```python
from build123d import *

# Parameters (mm, degrees)
SKETCH1_R                       = 72
SKETCH1_R_2                     = 60
BOSS_EXTRUDE1_DEPTH             = 25.4
BOSS_EXTRUDE4_DEPTH             = 12
CUT_EXTRUDE1_DEPTH              = 25.4
SKETCH8_W                       = 60
SKETCH8_H                       = 84.7705
BOSS_EXTRUDE5_DEPTH             = 12
CIRPATTERN4_COUNT               = 2
CIRPATTERN4_ANGLE               = 90
CIRPATTERN4_THE_OTHER_WAY_COUNT = 2
CIRPATTERN4_THE_OTHER_WAY_ANGLE = 90
M8_CLEARANCE_HOLE1_D            = 10
M8_CLEARANCE_HOLE1_DEPTH        = 12


with BuildPart() as part:
    # Sketch1 → Boss-Extrude1 (new body)
    with BuildSketch(Plane(origin=(0, 0, 0), x_dir=(1, 0, 0), z_dir=(0, 1, 0))):
        Circle(SKETCH1_R)
        Circle(SKETCH1_R_2, mode=Mode.SUBTRACT)
    extrude(amount=-BOSS_EXTRUDE1_DEPTH)

    # Sketch7 → Boss-Extrude4 (add)
    with BuildSketch(Plane(origin=(-60, 0, 0), x_dir=(0, 0, -1), z_dir=(1, 0, 0))):
        Polygon((-25, -25.4), (-25, -81.8336), (25, -81.8336), (25, -25.4), (25, 0), (-25, 0), align=None)
    extrude(amount=-BOSS_EXTRUDE4_DEPTH)

    # Sketch15 → Cut-Extrude1 (cut)
    with BuildSketch(Plane.XZ.offset(25.4)):
        Polygon((-60, 25), (-54.543560573, 25), (-54.543560573, -25), (-60, -25), (-60, 0), align=None)
    extrude(amount=-CUT_EXTRUDE1_DEPTH, mode=Mode.SUBTRACT)

    # Sketch8 → Boss-Extrude5 (add)
    with BuildSketch(Plane.ZY.offset(-60)):
        with Locations((0, -42.38525)):
            Rectangle(SKETCH8_W, SKETCH8_H)
    boss_extrude5 = extrude(amount=-BOSS_EXTRUDE5_DEPTH)

    # CirPattern4: Boss-Extrude5 ×2 about axis
    cirpattern4_axis = Axis((0, 0, 0), (0, 1, 0))
    for i in range(1, CIRPATTERN4_COUNT):
        add(boss_extrude5.rotate(cirpattern4_axis, i * CIRPATTERN4_ANGLE / (CIRPATTERN4_COUNT - 1)))

    # CirPattern4 the other way: Boss-Extrude5 ×2 about axis
    cirpattern4_the_other_way_axis = Axis((0, 0, 0), (0, -1, 0))
    for i in range(1, CIRPATTERN4_THE_OTHER_WAY_COUNT):
        add(boss_extrude5.rotate(cirpattern4_the_other_way_axis, i * CIRPATTERN4_THE_OTHER_WAY_ANGLE / (CIRPATTERN4_THE_OTHER_WAY_COUNT - 1)))

    # M8 Clearance Hole1
    with Locations(Plane.ZY.offset(-60)):
        with Locations((0, -59.7705)):
            Hole(M8_CLEARANCE_HOLE1_D / 2, depth=M8_CLEARANCE_HOLE1_DEPTH)


solid = part.part
```
Model file for the job. Use its own axes, mm. A direction names the side the tool comes from. Coordinates: 2 decimals unless noted, no trailing zeros. Write each loop counter-clockwise with the first axis right and the second up, starting at its lowest first coordinate (ties: lowest second). Pieces come first, ordered by that corner, then holes. Notation, with made-up numbers: (65, 57) - (101, 57) arc R35 ccw to (101, 91) - close; hole circle Ø3 at (53, 32.25). An arc over 180 degrees is marked (long way). One line per item, written item: value. Start each with the question number.
1. Slice it at C-C (z = 46.5). Write the cut outline in (x, y).
2. Slice it at A-A (y = -70.5). Write the cut outline in (x, z), plus the area to 3 significant figures.
3. Probe line 1 (Y direction, x = 69, z = 0); line 2 (X direction, y = -19, z = 0); line 3 (Z direction, x = -10.5, y = -22). List the from-to ranges inside material, lowest first. Write a range as from..to.
4. Flat gauge pins, fed straight in: pin 1 (20 mm diameter, centred on x = -39, z = 42, fed in from -Y); pin 2 (3 mm diameter, centred on y = -14, z = 38, fed in from -X); pin 3 (6 mm diameter, centred on x = -57.5, y = -7, fed in from -Z); pin 4 (2 mm diameter, centred on x = -17.5, z = 55, fed in from +Y). Where does each tip first touch, or does it go through?
5. Tool access for faces 1 (the flat face through (-30, -52, -66)), 2 (the flat face through (30, -52, -66)), 3 (the flat face through (30, -52, 66)): list every direction of +Z, -Z, +X, -X, +Y, -Y with a clear straight run to the whole face (end or side of a thin tool).
6. Slice it at D-D (z = -20). Write the cut outline in (x, y).
7. Slice it at B-B (x = 53). Write the cut outline in (y, z), plus the area to 3 significant figures.
8. Mould opens along X. For faces 4 (the flat face through (-60, -40, 0)), 5 (the flat face through (0, -84.77, 66)), 6 (the flat face through (-30, -52, 66)) say: released by +X, released by -X, zero draft, split by the parting line, or undercut.
Answers below:
1. outline: (-54.97, -25.4) - (-37.92, -25.4) - (-37.92, 0) - (-54.97, 0) - close; (37.92, -25.4) - (54.97, -25.4) - (54.97, 0) - (37.92, 0) - close
2. outline: (-72, -25) - (-60, -25) - (-60, 25) - (-72, 25) - close; (-30, -72) - (30, -72) - (30, -60) - (-30, -60) - close; (-30, 60) - (30, 60) - (30, 72) - (-30, 72) - close; (60, -30) - (72, -30) - (72, 30) - (60, 30) - close
2. area: 2,760 mm^2
3. line 1: y = -84.77..-64.77, -54.77..0
3. line 2: x = -72..-60, 60..72
3. line 3: z = -72..-59.07, 59.07..72
4. pin 1: stops at y = -25.4
4. pin 2: stops at x = -62.06
4. pin 3: stops at z = -47.05
4. pin 4: passes through
5. face 1: -Z, -X, -Y
5. face 2: -Z, +X, -Y
5. face 3: +Z, +X, -Y
6. outline: (-72, -81.83) - (-60, -81.83) - (-60, 0) - (-72, 0) - close; (56.57, -25.4) - (60, -25.4) - (60, -84.77) - (72, -84.77) - (72, 0) - (56.57, 0) - close
7. outline: (-25.4, -48.73) - (0, -48.73) - (0, -28.12) - (-25.4, -28.12) - close; (-25.4, 28.12) - (0, 28.12) - (0, 48.73) - (-25.4, 48.73) - close
7. area: 1,050 mm^2
8. face 4: undercut
8. face 5: zero draft
8. face 6: released by -X
